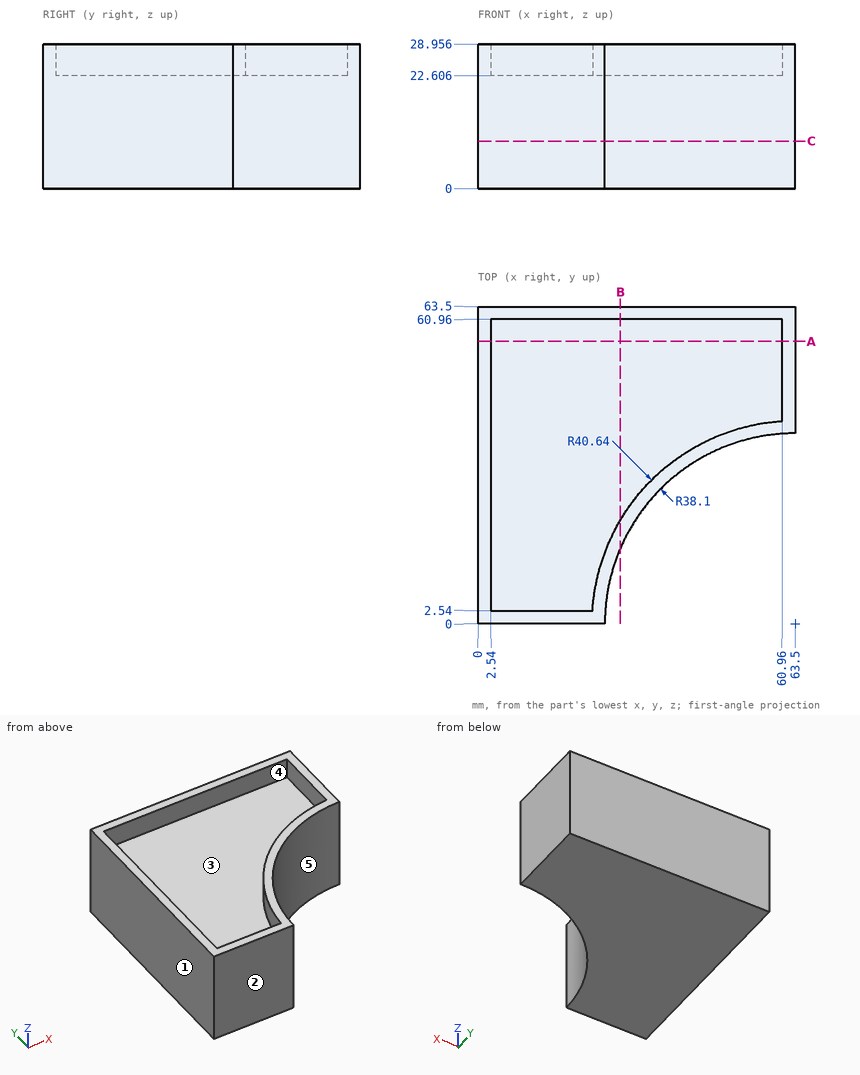
The figure shows three views and two pictorial views of one solid part (mm, origin at its lowest corner). Answer the questions. A direction names the side the tool comes from. Give positions to 0.01 mm unless a question says otherwise; leave off trailing zeros. Write each loop counter-clockwise with the first axis right and the second up, starting at its lowest first coordinate (ties: lowest second). Pieces come first, ordered by that corner, then holes. Notation, with made-up numbers: (27, 82.25) - (57, 82.25) arc R23 ccw to (57, 104.25) - close; hole circle Ø2 at (-28, -2.5). An arc over 180 degrees is marked (long way). Return JSON: item names as keys, results as strings.
Q1. Consider line 1 along X through (y, z) = (51, 25); line 2 along Z through (x, y) = (21, 60). Determine where each line is inside the solid, lowest interval first. Write a range as [from, to].
Reply:
{"line 1": "[0, 2.54], [60.96, 63.5]", "line 2": "[0, 22.61]"}
Q2. A cutting plane is placed at B-B, the plane x = 28.5. Determine the outline of the cut face in (y, z), and give its area (3 significant figures).
Reply:
{"outline": "(15.05, 0) - (63.5, 0) - (63.5, 28.96) - (60.96, 28.96) - (60.96, 22.61) - (20.65, 22.61) - (20.65, 28.96) - (15.05, 28.96) - close", "area": "1,150 mm²"}
Q3. A cutting plane is placed at A-A, the plane y = 56.5. Determine the outline of the cut face in (x, z), and give its area (3 significant figures).
Reply:
{"outline": "(0, 0) - (63.5, 0) - (63.5, 28.96) - (60.96, 28.96) - (60.96, 22.61) - (2.54, 22.61) - (2.54, 28.96) - (0, 28.96) - close", "area": "1,470 mm²"}
Q4. Given P1, Ø2, axis at x = 48.5, z = 15.5, coming from the -Y side; P2, Ø3, axis at y = 29.5, z = 26, coming from the +X side; P3, Ø10, axis at y = 10, z = 4, coming from the +X side, each flat-ended and moving along its own axis, determine where each tip first touches the part or whether it passes through.
Reply:
{"P1": "y = 34.58", "P2": "x = 41.35", "P3": "x = 28.48"}
Q5. For a pull along X with two mould halves and no side action, classify the marked faces 1, 2 and 3 as released by +X, released by -X, zero draft, split by the parting line, or undercut.
Reply:
{"face 1": "released by -X", "face 2": "zero draft", "face 3": "undercut"}
Q6. A cutting plane is placed at C-C, the plane z = 9.5. Determine the outline of the cut face in (x, y), and give its area (3 significant figures).
Reply:
{"outline": "(0, 0) - (25.4, 0) arc R38.1 cw to (63.5, 38.1) - (63.5, 63.5) - (0, 63.5) - close", "area": "2,890 mm²"}
Q7. For the marked faces 4 and 5, determine the directions among +Z, -Z, +X, -X, +Y, -Y from which every point of the face is accessible in a straight line to the end or side of a thin tool.
Reply:
{"face 4": "+Z", "face 5": "+Z, -Z, +X, -Y"}
